Autodesk Inventor part; units mm, degrees
ref_plane "YZ Plane" through (0, 0, 0) normal (1, 0, 0) x (0, 1, 0)
ref_plane "XZ Plane" through (0, 0, 0) normal (0, 1, 0) x (-1, 0, 0)
ref_plane "XY Plane" through (0, 0, 0) normal (0, 0, 1) x (1, 0, 0)
sketch "Sketch1" plane through (0, 0, 0) normal (0, 0, 1) x (1, 0, 0)
  line L0 (-25, -25) -> (25, -25)
  line L1 (25, -25) -> (25, 25)
  line L2 (25, 25) -> (5, 25)
  line L3 (-25, -25) -> (-25, -5)
  line L4 (-25, -5) -> (5, 25)
  point P0 (0, 0)
  dimension "d0" = 50
  dimension "d1" = 50
  dimension "d2" = 20
  dimension "d3" = 20
  dimension "d21" = 25
  dimension "d22" = 25
extrude "Extrusion1" add sketch "Sketch1" along normal blind 2.6568
sketch "Sketch2" plane through (0, 0, 2.6568) normal (0, 0, 1) x (1, 0, 0)
  line L0 (-25, -25) -> (25, -25)
  line L1 (25, -25) -> (25, 25)
  line L2 (-15, -15) -> (5, -15) construction
  line L3 (-15, -17.75) -> (5, -17.75)
  line L4 (5, -12.25) -> (-15, -12.25)
  arc A0 (-15, -12.25) -> (-15, -17.75) centre (-15, -15) ccw
  arc A1 (5, -17.75) -> (5, -12.25) centre (5, -15) ccw
  line L5 (15, -5) -> (15, 15) construction
  line L6 (17.75, -5) -> (17.75, 15)
  line L7 (12.25, 15) -> (12.25, -5)
  arc A2 (12.25, -5) -> (17.75, -5) centre (15, -5) ccw
  arc A3 (17.75, 15) -> (12.25, 15) centre (15, 15) ccw
  point P0 (0, 0)
  point P1 (-5, -15)
  point P2 (15, 5)
  dimension "d6" = 20
  dimension "d7" = 5.5
  dimension "d8" = 10
  dimension "d9" = 20
  dimension "d10" = 20
  dimension "d11" = 5.5
  dimension "d12" = 10
  dimension "d13" = 20
extrude "Extrusion2" cut sketch "Sketch2" against normal through all
sketch "Sketch3" plane through (0, 0, 2.6568) normal (0, 0, 1) x (1, 0, 0)
  line L0 (-25, -25) -> (25, -25)
  line L1 (25, -25) -> (25, 25)
  circle A0 centre (-5, 5) radius 3.302
  point P0 (0, 0)
  dimension "d16" = 6.604
  dimension "d17" = 30
  dimension "d18" = 30
extrude "Extrusion3" cut sketch "Sketch3" against normal through all
fillet "Fillet1" radius 2 5 edges at (-25, -25, 1.3284) (25, -25, 1.3284) (25, 25, 1.3284) (5, 25, 1.3284) (-25, -5, 1.3284)
equation "\"d0\" = d1"
properties part number "frame_gusset" material "Steel, Mild"
Can you work these out from the model? Positions are in its coordinate system, mm. A direction names the side the tool comes from. Give positions to 0.01 mm unless a question says otherwise; leave off trailing zeros. Write each loop counter-clockwise with the first axis right and the second up, starting at its lowest first coordinate (ties: lowest second). Pieces come first, ordered by that corner, then holes. Notation, with made-up numbers: (14.25, 64.5) -> (31.25, 64.5) arc R19 ccw to (31.25, 81.5) -> close; hole circle Ø6 at (-34, 32.5). An arc over 180 degrees is marked (long way). One line per item, written item: value.
Q1. Imagine slicing it at A-A on y = -15. Please give me the cut outline in (x, z), and give its area (3 significant figures).
Results found:
outline: (-25, 0) -> (-17.75, 0) -> (-17.75, 2.66) -> (-25, 2.66) -> close; (7.75, 0) -> (25, 0) -> (25, 2.66) -> (7.75, 2.66) -> close
area: 65.1 mm^2
Q2. Imagine slicing it at C-C on x = 15. Please give me the cut outline in (y, z), and give its area (3 significant figures).
Results found:
outline: (-25, 0) -> (-7.75, 0) -> (-7.75, 2.66) -> (-25, 2.66) -> close; (17.75, 0) -> (25, 0) -> (25, 2.66) -> (17.75, 2.66) -> close
area: 65.1 mm^2
Q3. We'd pull the mould along Y, two halves only. Please class faces 1 (the face through (17.75, 5, 1)), 2 (the face through (-10, 10, 1)), 3 (the face through (25, 0, 1)): +Y half, -Y half, draft (parallel to the pull), parting line (faces both ways), or undercut.
Results found:
face 1: undercut
face 2: +Y half
face 3: draft
Q4. Please list where these lines run through material, in increasing order: line 1 (Y direction, x = -5, z = 0.85); line 2 (Y direction, x = -4.5, z = 1.6); line 3 (X direction, y = -4, z = 1.75). Write a range as [from, to].
Results found:
line 1: y = [-25, -17.75], [-12.25, 1.7], [8.3, 15]
line 2: y = [-25, -17.75], [-12.25, 1.74], [8.26, 15.5]
line 3: x = [-24, 12.25], [17.75, 25]
Q5. Imagine slicing it at D-D on z = 1.2. Please give me the cut outline in (x, y).
Results found:
outline: (-25, -23) arc R2 ccw to (-23, -25) -> (23, -25) arc R2 ccw to (25, -23) -> (25, 23) arc R2 ccw to (23, 25) -> (5.83, 25) arc R2 ccw to (4.41, 24.41) -> (-24.41, -4.41) arc R2 ccw to (-25, -5.83) -> close; hole (-15, -17.75) -> (5, -17.75) arc R2.75 ccw to (5, -12.25) -> (-15, -12.25) arc R2.75 ccw to start; hole circle Ø6.6 at (-5, 5); hole (12.25, -5) arc R2.75 ccw to (17.75, -5) -> (17.75, 15) arc R2.75 ccw to (12.25, 15) -> close
Q6. Imagine slicing it at B-B on x = -5. Please give me the cut outline in (y, z), and give its area (3 significant figures).
Results found:
outline: (-25, 0) -> (-17.75, 0) -> (-17.75, 2.66) -> (-25, 2.66) -> close; (-12.25, 0) -> (1.7, 0) -> (1.7, 2.66) -> (-12.25, 2.66) -> close; (8.3, 0) -> (15, 0) -> (15, 2.66) -> (8.3, 2.66) -> close
area: 74.1 mm^2
Q7. Which directions (+Z, -Z, +X, -X, +Y, -Y) give clear straight access to the entire face, cutting with the end or side of a thin tool? Please do faces 4 (the face through (15.06, 17.75, 1.35)), 5 (the face through (24.4, -24.43, 1.35)).
Results found:
face 4: +Z, -Z
face 5: +Z, -Z, +X, -Y
Q8. For P1, Ø0.8, axis at y = 3.5, z = 1, coming from the -X side, with a flat end and sliding along its axis, tell me the tip position at first contact or that it passes through.
Results found:
P1: stops at x = -16.9
